Source: CAD feature listing. Evaluate the final solid. Frame: model axes, mm. Face numbers are marked on the shaded views. A direction names the side the tool comes from. Round coordinates to 2 decimals unless told otherwise and drop trailing zeros. Loops run counter-clockwise (first coordinate to the right, second up) from the corner with the lowest first, then second, coordinate; pieces in that order, holes last. Notation, with made-up numbers: (26.5, -31) -> (37.5, -31) arc R22 ccw to (37.5, -4) -> close; hole circle Ø2 at (-14, 26.25). An arc over 180 degrees is marked (long way). Write item = value, one per line.
from build123d import *

# Parameters (mm, degrees)
SKETCH1_R           = 1.25
BOSS_EXTRUDE1_DEPTH = 5
SKETCH2_W           = 20
SKETCH2_H           = 20
BOSS_EXTRUDE2_DEPTH = 17.8
SKETCH3_R           = 10
BOSS_EXTRUDE3_DEPTH = 40
CUT_EXTRUDE1_DEPTH  = 56.46025604
FILLET1_R           = 5
CHAMFER2_SIZE       = 3


with BuildPart() as part:
    # Sketch1 → Boss-Extrude1 (new body)
    with BuildSketch(Plane(origin=(0, 0, 0), x_dir=(1, 0, 0), z_dir=(0, 1, 0))):
        with BuildLine():
            Line((-10, -10), (10, -10))
            Line((10, -10), (10, -5))
            Line((10, -5), (15, -5))
            ThreePointArc((15, -5), (20, 0), (15, 5))
            Line((15, 5), (10, 5))
            Line((10, 5), (10, 10))
            Line((10, 10), (-10, 10))
            Line((-10, 10), (-10, 5))
            Line((-10, 5), (-15, 5))
            ThreePointArc((-15, 5), (-20, 0), (-15, -5))
            Line((-15, -5), (-10, -5))
            Line((-10, -5), (-10, -10))
        make_face()
        with Locations(Location((-15, 0, 0), (0, 0, 270))):
            Circle(SKETCH1_R, mode=Mode.SUBTRACT)
        with Locations(Location((15, 0, 0), (0, 0, 90))):
            Circle(SKETCH1_R, mode=Mode.SUBTRACT)
    extrude(amount=BOSS_EXTRUDE1_DEPTH)

    # Sketch2 → Boss-Extrude2 (add)
    with BuildSketch(Plane(origin=(0, 5, 0), x_dir=(1, 0, 0), z_dir=(0, 1, 0))):
        Rectangle(SKETCH2_W, SKETCH2_H)
    extrude(amount=BOSS_EXTRUDE2_DEPTH)

    # Sketch3 → Boss-Extrude3 (add)
    with BuildSketch(Plane(origin=(0, 0, -10), x_dir=(-1, 0, 0), z_dir=(0, 0, -1))):
        with Locations((0, 22.8)):
            Circle(SKETCH3_R)
    extrude(amount=-BOSS_EXTRUDE3_DEPTH)

    # Sketch3<3> → Cut-Extrude1 (cut, through all)
    with BuildSketch(Plane(origin=(0, 0, -10), x_dir=(-1, 0, 0), z_dir=(0, 0, -1))):
        with BuildLine():
            Line((-4.5, 22.8), (4.5, 22.8))
            ThreePointArc((4.5, 22.8), (0, 27.3), (-4.5, 22.8))
        make_face()
        with BuildLine():
            ThreePointArc((-4.5, 22.8), (0, 18.3), (4.5, 22.8))
            Line((4.5, 22.8), (-4.5, 22.8))
        make_face()
    extrude(amount=-CUT_EXTRUDE1_DEPTH, mode=Mode.SUBTRACT)

    # Fillet1
    fillet1_edges = [part.edges().sort_by_distance(p)[0] for p in [
        (10, 2.5, -5),
        (10, 2.5, 5),
        (-10, 2.5, 5),
        (-10, 2.5, -5),
    ]]
    fillet(fillet1_edges, radius=FILLET1_R - 0.0001)  # a hair under: the kernel refuses the full size

    # Chamfer2
    chamfer2_edges = [part.edges().sort_by_distance(p)[0] for p in [
        (4.5, 22.8, -10),
    ]]
    chamfer(chamfer2_edges, length=CHAMFER2_SIZE)


solid = part.part
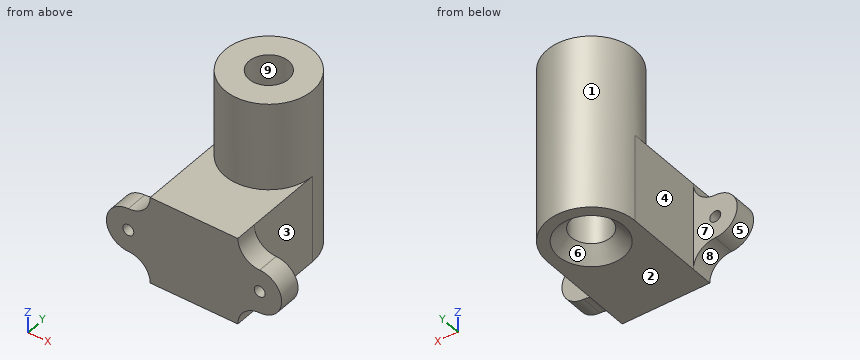
1. Contact query for flat-ended pins moving along their axis: pin 1 Ø1.5 at (y, z) = (10.5, -4) entering from -X; pin 2 Ø5 at (x, z) = (17, 4.5) entering from +Y; pin 3 Ø3 at (y, z) = (18, 16.5) entering from +X. Output: stop coordinate, or through.
Evaluation:
pin_1 = -10
pin_2 = 5
pin_3 = 9.44
2. Section query A-A (z = 0). Return the cut outline in (x, y), then the cut area to 3 significant figures.
Evaluation:
outline = (-20, 0) -> (-16.25, 0) -> (-16.25, 5) -> (-20, 5) -> close; (-13.75, 0) -> (13.75, 0) -> (13.75, 5) -> (10, 5) -> (10, 22.8) arc R10 ccw to (-10, 22.8) -> (-10, 5) -> (-13.75, 5) -> close; (16.25, 0) -> (20, 0) -> (20, 5) -> (16.25, 5) -> close; hole circle Ø9 at (0, 22.8)
area = 624 mm²
3. Section query B-B (y = 2). Give the number of separate pieces and of enclosed holes in the cut face, then the cut area to 3 significant figures.
Evaluation:
separate_pieces = 1
enclosed_holes = 2
area = 590 mm²
4. Line query: probe 1 along X at (y, z) = (3, 0); probe 2 along X at (y, z) = (22.8, 1); probe 3 along Y at (x, z) = (0, 13.5). Output: solid intervals per line, ascending. Write a range as from..to.
Evaluation:
probe_1 = -20..-16.25, -13.75..13.75, 16.25..20
probe_2 = -10..-4.5, 4.5..10
probe_3 = 12.8..18.3, 27.3..32.8
5. Mould query, pull axis X, two halves, no side actions, for the marked faces 6, 7, 8 and 9. Classes: released by +X, released by -X, zero draft, split by the parting line, or undercut.
Evaluation:
face_6 = undercut
face_7 = zero draft
face_8 = released by -X
face_9 = undercut
6. Section query C-C (x = 0). Return the cut outline in (y, z), then the cut area to 3 significant figures.
Evaluation:
outline = (0, -10) -> (15.3, -10) -> (18.3, -7) -> (18.3, 30) -> (12.8, 30) -> (12.8, 10) -> (0, 10) -> close; (27.3, -7) -> (30.3, -10) -> (32.8, -10) -> (32.8, 30) -> (27.3, 30) -> close
area = 687 mm²
7. Section query D-D (z = 19). Return the cut outline in (x, y), then the cut area to 3 significant figures.
Evaluation:
outline = circle Ø20 at (0, 22.8); hole circle Ø9 at (0, 22.8)
area = 251 mm²
8. Set-up query: the marked faces 1, 2, 3, 4 and 5. Return all of +Z, -Z, +X, -X, +Y, -Y with unobstructed straight access to the full face (end or side cutting, diameter ignored); none if empty.
Evaluation:
face_1 = +Z
face_2 = -Z, +X, -X, +Y, -Y
face_3 = +Z, -Z, +X, +Y
face_4 = +Z, -Z, -X, +Y
face_5 = -X, +Y, -Y
